from build123d import *

# Parameters (mm, degrees)
SKETCH1_W           = 13.75
SKETCH1_H           = 13.75
BOSS_EXTRUDE1_DEPTH = 10
SKETCH3_R           = 1.4
CUT_EXTRUDE1_DEPTH  = 19.339250939
SKETCH2_R           = 1.5
CUT_EXTRUDE2_DEPTH  = 14.947446003
FILLET1_R           = 1


with BuildPart() as part:
    # Sketch1 → Boss-Extrude1 (new body)
    with BuildSketch(Plane.XY):
        Rectangle(SKETCH1_W, SKETCH1_H)
    extrude(amount=BOSS_EXTRUDE1_DEPTH)

    # Sketch3 → Cut-Extrude1 (cut, through all)
    with BuildSketch(Plane(origin=(0, 6.875, 0), x_dir=(1, 0, 0), z_dir=(0, 1, 0))):
        with Locations(Location((0, -3, 0), (0, 0, 270))):
            Circle(SKETCH3_R)
    extrude(amount=-CUT_EXTRUDE1_DEPTH, mode=Mode.SUBTRACT)

    # Sketch2 → Cut-Extrude2 (cut, through all)
    with BuildSketch(Plane(origin=(0, 0, 0), x_dir=(-1, 0, 0), z_dir=(0, 0, -1))):
        with Locations((4, 0)):
            Circle(SKETCH2_R)
        with Locations((-4, 0)):
            Circle(SKETCH2_R)
    extrude(amount=-CUT_EXTRUDE2_DEPTH, mode=Mode.SUBTRACT)

    # Fillet1
    fillet1_edges = [part.edges().sort_by_distance(p)[0] for p in [
        (-6.875, 6.875, 5),
        (-6.875, -6.875, 5),
        (6.875, -6.875, 5),
        (6.875, 6.875, 5),
    ]]
    fillet(fillet1_edges, radius=FILLET1_R)


solid = part.part
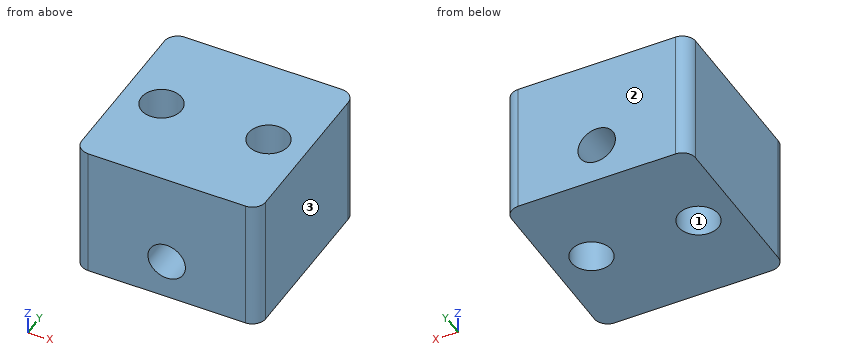
Input: part model. Units: mm. Frame: model coordinates. Face numbers are marked on the shaded views. Give positions to 0.01 mm unless a question says otherwise; leave off trailing zeros. Order: outer loops, then holes, each group sorted by start corner. A loop starts at its lowest first (then second) coordinate and runs counter-clockwise, first axis right, second up.
Q1. Ray query, probe 1 along Y at (x, z) = (-4, 2) (3 decimals); probe 2 along X at (y, z) = (-3.25, 3) (3 decimals); probe 3 along X at (y, z) = (-0.75, 3) (3 decimals). Return the intervals inside material, ascending.
Checked values:
probe 1: y = -6.875 to -1.5, 1.5 to 6.875
probe 2: x = -6.875 to -1.4, 1.4 to 6.875
probe 3: x = -6.875 to -5.299, -2.701 to -1.4, 1.4 to 2.701, 5.299 to 6.875
Q2. Section C-C on x = 0. Output: boundary loops of the cut face in (y, z) (3 decimals), and give its area (3 significant figures).
Checked values:
outline: (-6.875, 0) - (6.875, 0) - (6.875, 1.6) - (-6.875, 1.6) - close; (-6.875, 4.4) - (6.875, 4.4) - (6.875, 10) - (-6.875, 10) - close
area: 99.0 mm2
Q3. Section A-A on z = 3. Output: boundary loops of the cut face in (x, y) (3 decimals).
Checked values:
outline: (-6.875, -5.875) arc R1 ccw to (-5.875, -6.875) - (-1.4, -6.875) - (-1.4, 6.875) - (-5.875, 6.875) arc R1 ccw to (-6.875, 5.875) - close; (1.4, -6.875) - (5.875, -6.875) arc R1 ccw to (6.875, -5.875) - (6.875, 5.875) arc R1 ccw to (5.875, 6.875) - (1.4, 6.875) - close; hole circle Ø3 at (-4, 0); hole circle Ø3 at (4, 0)
Q4. Contact query for a flat-ended pin moving along its axis: pin 1 Ø2.5 at (x, y) = (-4, 0) entering from +Z. Output: stop coordinate, or through.
Checked values:
pin 1: passes through
Q5. Draft query along X for the marked faces 1, 2 and 3. Return one class per face: +X half, -X half, draft (parallel to the pull), parting line (faces both ways), or undercut.
Checked values:
face 1: undercut
face 2: draft
face 3: +X half
Q6. Section B-B on y = 0. Output: boundary loops of the cut face in (x, z) (3 decimals).
Checked values:
outline: (-6.875, 0) - (-5.5, 0) - (-5.5, 10) - (-6.875, 10) - close; (-2.5, 0) - (2.5, 0) - (2.5, 10) - (-2.5, 10) - close; (5.5, 0) - (6.875, 0) - (6.875, 10) - (5.5, 10) - close; hole circle Ø2.8 at (0, 3)
Q7. Section D-D on y = -3. Output: boundary loops of the cut face in (x, z) (3 decimals).
Checked values:
outline: (-6.875, 0) - (6.875, 0) - (6.875, 10) - (-6.875, 10) - close; hole circle Ø2.8 at (0, 3)
